```python
from build123d import *

# Parameters (mm, degrees)
F0_W        = 8
F0_H        = 3
F1_DEPTH    = 84
F3_D        = 4.3
F3_DEPTH    = 16
F3_START    = 5
F3_TIP      = 1.2918503309
F2_W        = 8
F2_H        = 64
F4_DEPTH    = 25
F5_R        = 3
F6_R        = 1
F7_T1_DEPTH = 101.4328702047


# Not quite as in the source:
# - a fillet or chamfer that OpenCascade refuses, or shapes differently, is made with other operations: its cross-section is extruded or revolved along the edge and cut away or added


with BuildPart() as f1:
    # F0 (on Top) → F1 (new body)
    with BuildSketch(Plane.XY):
        with Locations((-12, -6.5)):
            Rectangle(F0_W, F0_H)
        with BuildLine():
            ThreePointArc((0, -8), (-5.6568542495, -5.6568542495), (-8, 0))
            Line((-8, 0), (-8, -5))
            Line((-8, -5), (-8, -8))
            Line((-8, -8), (-2.5, -8))
            Line((-2.5, -8), (0, -8))
        make_face()
        with BuildLine():
            ThreePointArc((2.4590163934, 5.4729551777), (0, -6), (-2.4590163934, 5.4729551777))
            Line((-2.4590163934, 5.4729551777), (-2.5, 7.5993420768))
            ThreePointArc((-2.5, 7.5993420768), (-6.4807406984, 4.6904157598), (-8, 0))
            ThreePointArc((-8, 0), (-5.6568542495, -5.6568542495), (0, -8))
            ThreePointArc((0, -8), (5.6568542495, -5.6568542495), (8, 0))
            ThreePointArc((8, 0), (6.4807406984, 4.6904157598), (2.5, 7.5993420768))
            Line((2.5, 7.5993420768), (2.4590163934, 5.4729551777))
        make_face()
        with BuildLine():
            Line((8, -5), (8, 0))
            ThreePointArc((8, 0), (5.6568542495, -5.6568542495), (0, -8))
            Line((0, -8), (2.5, -8))
            Line((2.5, -8), (8, -8))
            Line((8, -8), (8, -5))
        make_face()
        with Locations((12, -6.5)):
            Rectangle(F0_W, F0_H)
    extrude(amount=F1_DEPTH)

    # F3
    # its depths count from where the whole tool has entered the part; down to there all is cleared
    with Locations(Plane(origin=(0, 0, 0), x_dir=(1, 0, 0), z_dir=(0, 1, 0)).offset(-F3_START)):
        with Locations((12, -5), (-12, -5), (12, -79), (-12, -79)):
            Hole(F3_D / 2, depth=F3_DEPTH)
            with Locations((0, 0, -(F3_DEPTH + F3_TIP / 2))):  # 118° drill point
                Cone(0, F3_D / 2, F3_TIP, mode=Mode.SUBTRACT)

    # F2 (on Front) → F4 (cut)
    with BuildSketch(Plane.XZ):
        with Locations((12, 42)):
            Rectangle(F2_W, F2_H)
        with Locations((-12, 42)):
            Rectangle(F2_W, F2_H)
    extrude(amount=F4_DEPTH, mode=Mode.SUBTRACT)

    # F5
    f5_edges = [f1.edges().sort_by_distance(p)[0] for p in [
        (-16, -6.5, 84),
        (-16, -6.5, 74),
        (16, -6.5, 84),
        (16, -6.5, 74),
        (-16, -6.5, 0),
        (16, -6.5, 0),
        (16, -6.5, 10),
        (-16, -6.5, 10),
        (-8, -6.5, 10),
        (8, -6.5, 10),
        (-8, -6.5, 74),
        (8, -6.5, 74),
    ]]
    fillet(f5_edges, radius=F5_R)

    # F6
    f6_edges = [f1.edges().sort_by_distance(p)[0] for p in [
        (-8, -5, 5),
        (8, -5, 5),
        (8, -5, 79),
        (-8, -5, 79),
    ]]
    fillet(f6_edges, radius=F6_R)

    # F7: fillet of radius 2 on 2 edges, made by hand

    # F7_s2 → F7_t1 (cut)
    with BuildSketch(Plane.XY.offset(-8.7164351024)):
        with BuildLine():
            ThreePointArc((2.4590163934, 5.4729551777), (3.8977705539, 6.3481743906), (5.4949420866, 5.8142593221))
            ThreePointArc((5.4949420866, 5.8142593221), (4.0959009817, 6.8719426036), (2.5, 7.5993420768))
            Line((2.5, 7.5993420768), (2.4590163934, 5.4729551777))
        make_face()
        with BuildLine():
            ThreePointArc((-5.4949420866, 5.8142593221), (-3.8977705539, 6.3481743906), (-2.4590163934, 5.4729551777))
            Line((-2.4590163934, 5.4729551777), (-2.5, 7.5993420768))
            ThreePointArc((-2.5, 7.5993420768), (-4.0959009817, 6.8719426036), (-5.4949420866, 5.8142593221))
        make_face()
    extrude(amount=F7_T1_DEPTH, mode=Mode.SUBTRACT)


solid = f1.part
```
Geometry: final body of the model. Coordinates: model frame, mm. A direction names the side the tool comes from. Round coordinates to 2 decimals unless told otherwise and drop trailing zeros. Write each loop counter-clockwise with the first axis right and the second up, starting at its lowest first coordinate (ties: lowest second). Pieces come first, ordered by that corner, then holes.
Item 1: Section query D-D (z = 49). Return loops of the section in (x, y), plus the area to 3 significant figures.
Item 2: Section query C-C (y = -1). Return loops of the section in (x, z), plus the area to 3 significant figures.
Item 3: Material intervals for L1, parallel to X at y = -6.75, z = 79; L2, parallel to Z at x = -12, y = -7.3; L3, parallel to Y at x = 0, z = 55, sorted ascending.
Item 4: Pin query (flat end, axial travel): P1, Ø2, axis at x = 3, z = 18, coming from the +Y side; P2, Ø4, axis at x = 11, z = 24.5, coming from the +Y side; P3, Ø7.5, axis at x = -13, z = 77, coming from the +Y side; P4, Ø5, axis at y = -0.5, z = 39, coming from the -X side. Return the tip coordinate at first contact, or that it passes through.
Item 5: Section query B-B (x = -12). Return loops of the section in (y, z), plus the area to 3 significant figures.
Item 6: Mould query, pull axis X, two halves, no side actions, for faces 4 (the face through (11.01, -6.52, 6.91)), 5 (the face through (-12.99, -6.52, 80.91)), 6 (the face through (0, -8, 41)), 7 (the face through (-15.14, -6.48, 83.1)). Classes: +X half, -X half, draft (parallel to the pull), parting line (faces both ways), or undercut.
Item 7: Section query A-A (z = 5). Return loops of the section in (x, y).
Item 8: Set-up query: faces 1 (the face through (-13.3, -5, 2.9)), 2 (the face through (12, -6, 74)), 3 (the face through (14, -5, 77)). Return all of +Z, -Z, +X, -X, +Y, -Y with unobstructed straight access to the full face (end or side cutting, diameter ignored); none if empty.
Completed:
1. outline: (-8, -8) - (8, -8) - (8, 0) arc R8 ccw to (5.49, 5.81) arc R2 ccw to (2.46, 5.47) arc R6 cw (long way) to (-2.46, 5.47) arc R2 ccw to (-5.49, 5.81) arc R8 ccw to (-8, 0) - close
1. area: 101 mm2
2. outline: (-8, 0) - (-5.92, 0) - (-5.92, 84) - (-8, 84) - close; (5.92, 0) - (8, 0) - (8, 84) - (5.92, 84) - close
2. area: 350 mm2
3. L1: x = -16 to -14.15, -9.85 to 9.85, 14.15 to 16
3. L2: z = 0 to 2.85, 7.15 to 10, 74 to 76.85, 81.15 to 84
3. L3: y = -8 to -6
4. P1: stops at y = 6.36
4. P2: passes through
4. P3: stops at y = -5
4. P4: stops at x = -8
5. outline: (-8, 0) - (-5, 0) - (-5, 2.85) - (-8, 2.85) - close; (-8, 7.15) - (-5, 7.15) - (-5, 10) - (-8, 10) - close; (-8, 74) - (-5, 74) - (-5, 76.85) - (-8, 76.85) - close; (-8, 81.15) - (-5, 81.15) - (-5, 84) - (-8, 84) - close
5. area: 34.2 mm2
6. face 4: undercut
6. face 5: undercut
6. face 6: draft
6. face 7: -X half
7. outline: (-16, -8) - (-14.15, -8) - (-14.15, -5) - (-16, -5) - close; (-9.85, -8) - (9.85, -8) - (9.85, -5) - (9, -5) arc R1 cw to (8, -4) - (8, 0) arc R8 ccw to (5.49, 5.81) arc R2 ccw to (2.46, 5.47) arc R6 cw (long way) to (-2.46, 5.47) arc R2 ccw to (-5.49, 5.81) arc R8 ccw to (-8, 0) - (-8, -4) arc R1 cw to (-9, -5) - (-9.85, -5) - close; (14.15, -8) - (16, -8) - (16, -5) - (14.15, -5) - close
8. face 1: +Z, -Z, -X, +Y
8. face 2: +X, +Y, -Y
8. face 3: +Z, -Z, +X, +Y
